Drawing for the job (mm, zero at the part's lowest x, y, z). A direction names the side the tool comes from. Give positions to 0.01 mm unless a question says otherwise; leave off trailing zeros. Loops run counter-clockwise (first coordinate to the right, second up) from the corner with the lowest first, then second, coordinate; pieces in that order, holes last. Notation, with made-up numbers: M -14,55 L 14,55 A18 cw 14,86 Z; hole C 87.25,64 d9. An arc over 180 degrees is marked long. Use CSV: the item, a comma, the result in double quotes. Start each with the question number.
(1) Slice it at D-D on z = 5. List the corners of the cut face in (x, y), and give its area (3 significant figures).
(2) Wall check: line 1 along Y through (x, z) = (5.5, 6.75); line 2 along Z through (x, y) = (10, 0.75); line 3 along X through (y, z) = (2.75, 1). Give the ranges that are in metal, low to high. Write a range as from..to.
(3) Two-plate mould, pull along Z, no slides. Class the marked faces 1, 2 and 3: pulls with the +Z half, pulls with the -Z half, needs draft (parallel to the pull), parting line crosses it, or undercut.
(4) Slice it at A-A on x = 10.25. List the corners of the cut face in (y, z).
(5) Flat gauge pin, fed straight in: P1, Ø3, axis at x = 11, y = 1, coming from the -Z side. Where does the tip first touch, or does it go through?
(6) Tool access for the marked faces 4, 5 and 6: list every direction of +Z, -Z, +X, -X, +Y, -Y with a clear straight run to the whole face (end or side of a thin tool).
(7) Slice it at C-C on x = 14.25. List the corners of the cut face in (y, z).
(8) Slice it at B-B on y = 2.25. List the corners of the cut face in (x, z), and give its area (3 significant figures).
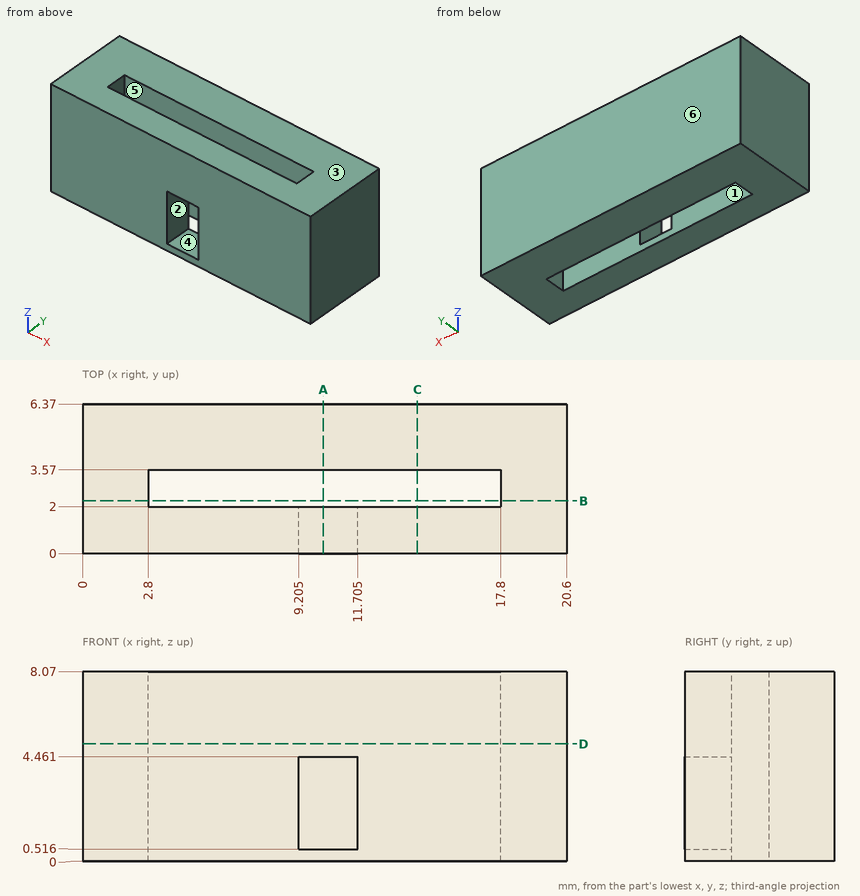
Reply:
1,outline,"M 0,0 L 20.6,0 L 20.6,6.37 L 0,6.37 Z; hole M 2.8,2 L 17.8,2 L 17.8,3.57 L 2.8,3.57 Z"
1,area,"108 mm^2"
2,line 1,"y = 0..2, 3.57..6.37"
2,line 2,"z = 0..0.52, 4.46..8.07"
2,line 3,"x = 0..2.8, 17.8..20.6"
3,face 1,"needs draft"
3,face 2,"undercut"
3,face 3,"pulls with the +Z half"
4,outline,"M 0,0 L 2,0 L 2,0.52 L 0,0.52 Z; M 0,4.46 L 2,4.46 L 2,8.07 L 0,8.07 Z; M 3.57,0 L 6.37,0 L 6.37,8.07 L 3.57,8.07 Z"
5,P1,"stops at z = 0"
6,face 4,"-Y"
6,face 5,"+Z, -Z"
6,face 6,"+Z, -Z, +X, -X, +Y"
7,outline,"M 0,0 L 2,0 L 2,8.07 L 0,8.07 Z; M 3.57,0 L 6.37,0 L 6.37,8.07 L 3.57,8.07 Z"
8,outline,"M 0,0 L 2.8,0 L 2.8,8.07 L 0,8.07 Z; M 17.8,0 L 20.6,0 L 20.6,8.07 L 17.8,8.07 Z"
8,area,"45.2 mm^2"
